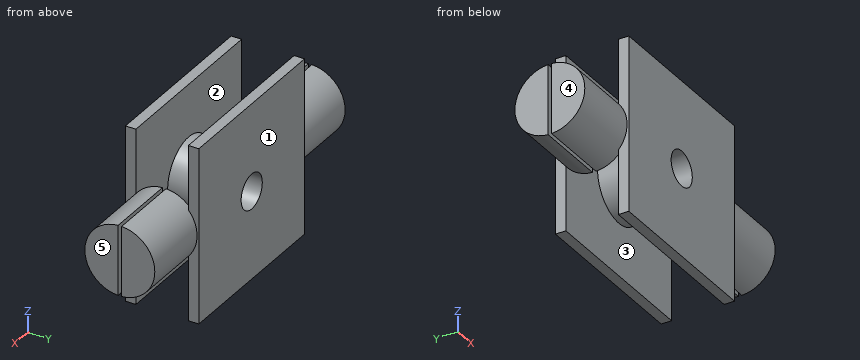
```python
from build123d import *

# Parameters (mm, degrees)
SKETCH1_R                = 10
BOSS_EXTRUDE1_DEPTH      = 15
SKETCH3_W                = 50
SKETCH3_H                = 50
BOSS_EXTRUDE2_DEPTH      = 3
SKETCH5_W                = 50
SKETCH5_H                = 50
BOSS_EXTRUDE4_DEPTH      = 3
SKETCH7_R                = 10
BOSS_EXTRUDE5_DEPTH      = 20
BOSS_EXTRUDE5_DEPTH_BACK = 1
SKETCH8_R                = 10
BOSS_EXTRUDE6_DEPTH      = 20
BOSS_EXTRUDE6_DEPTH_BACK = 1
SKETCH9_W                = 28.965508976
SKETCH9_H                = 1
CUT_EXTRUDE2_DEPTH       = 21
SKETCH10_W               = 34.685430092
SKETCH10_H               = 1
CUT_EXTRUDE3_DEPTH       = 21
SKETCH6_R                = 5
CUT_EXTRUDE4_DEPTH       = 56.596762496
CUT_EXTRUDE5_START       = -2
SKETCH11_R               = 8
CUT_EXTRUDE5_DEPTH       = 17


with BuildPart() as part:
    # Sketch1 → Boss-Extrude1 (new body)
    with BuildSketch(Plane(origin=(0, 0, 0), x_dir=(1, 0, 0), z_dir=(0, 1, 0))):
        with Locations(Location((0, 0, 0), (0, 0, 270))):
            Circle(SKETCH1_R)
    extrude(amount=BOSS_EXTRUDE1_DEPTH)

    # Sketch3 → Boss-Extrude2 (add)
    with BuildSketch(Plane.XZ):
        Rectangle(SKETCH3_W, SKETCH3_H)
    extrude(amount=BOSS_EXTRUDE2_DEPTH)

    # Sketch5 → Boss-Extrude4 (add)
    with BuildSketch(Plane(origin=(0, 15, 0), x_dir=(1, 0, 0), z_dir=(0, 1, 0))):
        Rectangle(SKETCH5_W, SKETCH5_H)
    extrude(amount=BOSS_EXTRUDE4_DEPTH)

    # Sketch7 → Boss-Extrude5 (add, two sides)
    with BuildSketch(Plane.ZY.offset(25)) as boss_extrude5_sk:
        with Locations((0, 7.5)):
            Circle(SKETCH7_R)
    extrude(amount=BOSS_EXTRUDE5_DEPTH)
    extrude(boss_extrude5_sk.sketch, amount=-BOSS_EXTRUDE5_DEPTH_BACK)

    # Sketch8 → Boss-Extrude6 (add, two sides)
    with BuildSketch(Plane(origin=(25, 0, 0), x_dir=(0, 0, -1), z_dir=(1, 0, 0))) as boss_extrude6_sk:
        with Locations(Location((0, 7.5, 0), (0, 0, 180))):
            Circle(SKETCH8_R)
    extrude(amount=BOSS_EXTRUDE6_DEPTH)
    extrude(boss_extrude6_sk.sketch, amount=-BOSS_EXTRUDE6_DEPTH_BACK)

    # Sketch9 → Cut-Extrude2 (cut)
    with BuildSketch(Plane.ZY.offset(45)):
        with Locations((0, 7.5)):
            Rectangle(SKETCH9_W, SKETCH9_H)
    extrude(amount=-CUT_EXTRUDE2_DEPTH, mode=Mode.SUBTRACT)

    # Sketch10 → Cut-Extrude3 (cut)
    with BuildSketch(Plane(origin=(45, 0, 0), x_dir=(0, 0, -1), z_dir=(1, 0, 0))):
        with Locations((0, 7.5)):
            Rectangle(SKETCH10_W, SKETCH10_H)
    extrude(amount=-CUT_EXTRUDE3_DEPTH, mode=Mode.SUBTRACT)

    # Sketch6 → Cut-Extrude4 (cut, through all)
    with BuildSketch(Plane(origin=(0, 18, 0), x_dir=(1, 0, 0), z_dir=(0, 1, 0))):
        with Locations(Location((0, 0, 0), (0, 0, 270))):
            Circle(SKETCH6_R)
    extrude(amount=-CUT_EXTRUDE4_DEPTH, mode=Mode.SUBTRACT)

    # Sketch11 → Cut-Extrude5 (cut)
    with BuildSketch(Plane.ZY.offset(45).offset(CUT_EXTRUDE5_START)):
        with Locations((0, 7.5)):
            Circle(SKETCH11_R)
    extrude(amount=-CUT_EXTRUDE5_DEPTH, mode=Mode.SUBTRACT)

    # SurfaceCut1
    split(bisect_by=Plane(origin=(0, 0, 0), x_dir=(0, 0, -1), z_dir=(1, 0, 0)), keep=Keep.BOTTOM)

    # Mirror2: part across plane


with BuildPart() as part_1:
    add(part.part)
    add(part.part.mirror(Plane(origin=(0, 0, 0), x_dir=(0, 0, 1), z_dir=(1, 0, 0))))


solid = part_1.part
```
Can you work these out from the model? Positions are in its coordinate system, mm. Face numbers are marked on the shaded views. A direction names the side the tool comes from. Round coordinates to 2 decimals unless told otherwise and drop trailing zeros. Loops run counter-clockwise (first coordinate to the right, second up) from the corner with the lowest first, then second, coordinate; pieces in that order, holes last. Notation, with made-up numbers: M -6,-16.75 L 36,-16.75 A19 cw 36,-2.75 Z; hole C 61,-37.5 d4. An arc over 180 degrees is marked long. Answer in a Markdown table with one row per item.
1. Please list where these lines run through material, in increasing order: line 1 (X direction, y = 13.5, z = 0); line 2 (Y direction, x = 5.5, z = 10); line 3 (X direction, y = 9.25, z = -2.5). Write a range as from..to.
Established:
| item | result |
|---|---|
| line 1 | -45..-43, -26..-24, -10..-5, 5..10, 24..26, 43..45 |
| line 2 | -3..0, 15..18 |
| line 3 | -45..-43, -26..-24, -9.68..-4.33, 4.33..9.68, 24..26, 43..45 |
2. If we section it at B-B, the plane z = 19: Please give me the cut outline in (x, y), plus the area to 3 significant figures.
Established:
| item | result |
|---|---|
| outline | M -25,-3 L 25,-3 L 25,0 L -25,0 Z; M -25,15 L 25,15 L 25,18 L -25,18 Z |
| area | 300 mm² |
3. If we section it at D-D, the plane z = -9: Please give me the cut outline in (x, y), plus the area to 3 significant figures.
Established:
| item | result |
|---|---|
| outline | M -45,3.14 L -24,3.14 L -24,7 L -45,7 Z; M -45,8 L -24,8 L -24,11.86 L -45,11.86 Z; M -25,-3 L 25,-3 L 25,0 L 4.36,0 L 4.36,15 L 25,15 L 25,18 L -25,18 L -25,15 L -4.36,15 L -4.36,0 L -25,0 Z; M 24,3.14 L 45,3.14 L 45,7 L 24,7 Z; M 24,8 L 45,8 L 45,11.86 L 24,11.86 Z |
| area | 755 mm² |
4. Thinking about a two-plate mould opening in X: for the marked faces 3, 4 and 5, which applies, pulls with the +X half, pulls with the -X half, needs draft (parallel to the pull), parting line crosses it, or undercut?
Established:
| item | result |
|---|---|
| face 3 | undercut |
| face 4 | pulls with the -X half |
| face 5 | pulls with the +X half |
5. If we section it at A-A, the plane x = 0: Please give me the cut outline in (y, z), plus the area to 3 significant figures.
Established:
| item | result |
|---|---|
| outline | M -3,-25 L 0,-25 L 0,-10 L 15,-10 L 15,-25 L 18,-25 L 18,-5 L -3,-5 Z; M -3,5 L 18,5 L 18,25 L 15,25 L 15,10 L 0,10 L 0,25 L -3,25 Z |
| area | 390 mm² |
6. I'm going to push flat-ended pins straight in: pin 1 Ø10 at (x, z) = (-33, 4.5) entering from -Y; pin 2 Ø0.9 at (y, z) = (-1.5, 10) entering from +X; pin 3 Ø5 at (x, y) = (-29.5, 3) entering from -Z; pin 4 Ø12 at (x, z) = (-2, -2) entering from +Y. Where does each tip first touch, or does it pass through?
Established:
| item | result |
|---|---|
| pin 1 | y = -2.5 |
| pin 2 | x = 25 |
| pin 3 | z = -9.8 |
| pin 4 | y = 18 |
7. On a 3-axis mill with a long thin cutter (end or side, diameter ignored), from which of +Z, -Z, +X, -X, +Y, -Y can I reach the whole of each face in a straight line? I mean the marked faces 1 and 2. Say none if no direction works.
Established:
| item | result |
|---|---|
| face 1 | +Z, -Z, +X, -X, +Y |
| face 2 | none |
